```python
from build123d import *

# Parameters (mm, degrees)
BOSS_EXTRUDE1_DEPTH = 20
SKETCH2_R           = 4.835
BOSS_EXTRUDE2_DEPTH = 4
CUT_EXTRUDE1_REACH  = 64.738
SKETCH3_R           = 7.665
CUT_EXTRUDE2_DEPTH  = 10
SKETCH5_W           = 6
SKETCH5_H           = 4
CUT_EXTRUDE3_DEPTH  = 10
CUT_EXTRUDE4_REACH  = 64.738
SKETCH6_R           = 1.165
BOSS_EXTRUDE4_DEPTH = 4
BOSS_EXTRUDE5_START = -4
BOSS_EXTRUDE5_DEPTH = 4
CHAMFER1_SIZE       = 3
CHAMFER2_SIZE       = 1
CHAMFER3_SIZE       = 1


with BuildPart() as part:
    # Sketch1 → Boss-Extrude1 (new body)
    with BuildSketch(Plane.XY):
        Polygon((-40.25, -10), (-40.25, -6), (-50, -6), (-56, -6), (-56, 6), (-50, 6), (-40.25, 6), (-40.25, 10), (0, 10), (2.25, 10), (2.25, 6), (0, 6), (-9.75, 6), (-9.75, -6), (0, -6), (2.25, -6), (2.25, -10), (0, -10), align=None)
    extrude(amount=BOSS_EXTRUDE1_DEPTH)

    # Sketch2 → Boss-Extrude2 (add)
    with BuildSketch(Plane.XZ.offset(6)):
        with Locations(Location((-50, 10, 0), (0, 0, 180))):
            Circle(SKETCH2_R)
    boss_extrude2 = extrude(amount=BOSS_EXTRUDE2_DEPTH)

    # Cut-Extrude1: up to this face of the body (flat: up to its plane)
    cut_extrude1_end = Plane(part.part.faces().sort_by_distance((-19, 10, 10))[0])
    # Sketch3 → Cut-Extrude1 (cut, up to the picked face)
    with BuildSketch(Plane.XZ.offset(10), mode=Mode.PRIVATE) as cut_extrude1_sk1:
        with Locations((0, 10)):
            Circle(SKETCH3_R)
    cut_extrude1_tool1 = split(extrude(cut_extrude1_sk1.sketch, amount=-CUT_EXTRUDE1_REACH, mode=Mode.PRIVATE), bisect_by=cut_extrude1_end, keep=Keep.BOTH, mode=Mode.PRIVATE)
    add(cut_extrude1_tool1.solids().sort_by(Axis((0, -10, 10), (0, 1, 0)))[0], mode=Mode.SUBTRACT)

    # Mirror1: Boss-Extrude2 across plane
    add(boss_extrude2.mirror(Plane.ZX))

    # Sketch4 → Cut-Extrude2 (cut)
    with BuildSketch(Plane.XY.offset(20)):
        Polygon((-27.5, 2.5), (-22.5, 2.062556682), (-22.5, -2.062556682), (-27.5, -2.5), align=None)
    extrude(amount=-CUT_EXTRUDE2_DEPTH, mode=Mode.SUBTRACT)

    # Sketch5 → Cut-Extrude3 (cut)
    with BuildSketch(Plane.XY.offset(20)):
        with Locations((-30.5, 5.165)):
            Rectangle(SKETCH5_W, SKETCH5_H)
        with Locations((-19.5, 5.165)):
            Rectangle(SKETCH5_W, SKETCH5_H)
        with Locations((-19.5, -5.165)):
            Rectangle(SKETCH5_W, SKETCH5_H)
        with Locations((-30.5, -5.165)):
            Rectangle(SKETCH5_W, SKETCH5_H)
    extrude(amount=-CUT_EXTRUDE3_DEPTH, mode=Mode.SUBTRACT)

    # Cut-Extrude4: up to this face of the body (flat: up to its plane)
    cut_extrude4_end = Plane(part.part.faces().sort_by_distance((-21.952820108, 10, 10))[0])
    # Sketch6 → Cut-Extrude4 (cut, up to the picked face)
    with BuildSketch(Plane.XZ.offset(10), mode=Mode.PRIVATE) as cut_extrude4_sk1:
        with Locations(Location((-30.5, 13, 0), (0, 0, 270))):
            Circle(SKETCH6_R)
    cut_extrude4_tool1 = split(extrude(cut_extrude4_sk1.sketch, amount=-CUT_EXTRUDE4_REACH, mode=Mode.PRIVATE), bisect_by=cut_extrude4_end, keep=Keep.BOTH, mode=Mode.PRIVATE)
    # Sketch6 → Cut-Extrude4 (cut, up to the picked face)
    with BuildSketch(Plane.XZ.offset(10), mode=Mode.PRIVATE) as cut_extrude4_sk2:
        with Locations((-25, 13)):
            Circle(SKETCH6_R)
    cut_extrude4_tool2 = split(extrude(cut_extrude4_sk2.sketch, amount=-CUT_EXTRUDE4_REACH, mode=Mode.PRIVATE), bisect_by=cut_extrude4_end, keep=Keep.BOTH, mode=Mode.PRIVATE)
    # Sketch6 → Cut-Extrude4 (cut, up to the picked face)
    with BuildSketch(Plane.XZ.offset(10), mode=Mode.PRIVATE) as cut_extrude4_sk3:
        with Locations(Location((-19.5, 13, 0), (0, 0, 90))):
            Circle(SKETCH6_R)
    cut_extrude4_tool3 = split(extrude(cut_extrude4_sk3.sketch, amount=-CUT_EXTRUDE4_REACH, mode=Mode.PRIVATE), bisect_by=cut_extrude4_end, keep=Keep.BOTH, mode=Mode.PRIVATE)
    add(cut_extrude4_tool1.solids().sort_by(Axis((-30.5, -10, 13), (0, 1, 0)))[0], mode=Mode.SUBTRACT)
    add(cut_extrude4_tool2.solids().sort_by(Axis((-25, -10, 13), (0, 1, 0)))[0], mode=Mode.SUBTRACT)
    add(cut_extrude4_tool3.solids().sort_by(Axis((-19.5, -10, 13), (0, 1, 0)))[0], mode=Mode.SUBTRACT)

    # Sketch10 → Boss-Extrude4 (add)
    with BuildSketch(Plane.XZ.offset(10)):
        with BuildLine():
            Line((2.25, 17.327327275), (3.717710372, 22.107058049))
            ThreePointArc((3.717710372, 22.107058049), (-12.665, 10), (3.717710372, -2.107058049))
            Line((3.717710372, -2.107058049), (2.25, 2.672672725))
            ThreePointArc((2.25, 2.672672725), (-7.665, 10), (2.25, 17.327327275))
        make_face()
    extrude(amount=-BOSS_EXTRUDE4_DEPTH)

    # Sketch11 → Boss-Extrude5 (add)
    with BuildSketch(Plane(origin=(0, 10, 0), x_dir=(1, 0, 0), z_dir=(0, 1, 0)).offset(BOSS_EXTRUDE5_START)):
        with BuildLine():
            Line((-9.75, -20), (-7.771886837, -20))
            ThreePointArc((-7.771886837, -20), (-2.284515289, -22.457255512), (3.717710372, -22.107058049))
            Line((3.717710372, -22.107058049), (2.25, -17.327327275))
            ThreePointArc((2.25, -17.327327275), (-7.665, -10), (2.25, -2.672672725))
            Line((2.25, -2.672672725), (3.717710372, 2.107058049))
            ThreePointArc((3.717710372, 2.107058049), (-2.284515289, 2.457255512), (-7.771886837, 0))
            Line((-7.771886837, 0), (-9.75, 0))
            Line((-9.75, 0), (-9.75, -20))
        make_face()
    extrude(amount=BOSS_EXTRUDE5_DEPTH)

    # Chamfer1
    # the kernel refuses this chamfer: 3 mm, written as the material it takes off along each edge
    with BuildSketch(Plane(origin=(-30.5, -10, 13), x_dir=(0, 0, -1), z_dir=(-1, 0, 0))) as chamfer1_piece_1:
        Polygon((1.165, -CHAMFER1_SIZE), (1.165 + CHAMFER1_SIZE, 0), (1.165, 0), align=None)
    revolve(axis=Axis((-30.5, -10, 13), (0, -1, 0)), mode=Mode.SUBTRACT)
    with BuildSketch(Plane(origin=(-25, -10, 13), x_dir=(1, 0, 0), z_dir=(0, 0, -1))) as chamfer1_piece_2:
        Polygon((1.165, -CHAMFER1_SIZE), (1.165 + CHAMFER1_SIZE, 0), (1.165, 0), align=None)
    revolve(axis=Axis((-25, -10, 13), (0, -1, 0)), mode=Mode.SUBTRACT)
    with BuildSketch(Plane(origin=(-19.5, -10, 13), x_dir=(0, 0, 1), z_dir=(1, 0, 0))) as chamfer1_piece_3:
        Polygon((1.165, -CHAMFER1_SIZE), (1.165 + CHAMFER1_SIZE, 0), (1.165, 0), align=None)
    revolve(axis=Axis((-19.5, -10, 13), (0, -1, 0)), mode=Mode.SUBTRACT)

    # Chamfer2
    chamfer2_edges = [part.edges().sort_by_distance(p)[0] for p in [
        (-45.165, -10, 10),
    ]]
    chamfer(chamfer2_edges, length=CHAMFER2_SIZE)

    # Chamfer3
    chamfer3_edges = [part.edges().sort_by_distance(p)[0] for p in [
        (-45.165, 10, 10),
    ]]
    chamfer(chamfer3_edges, length=CHAMFER3_SIZE)


solid = part.part
```
Check sheet for the modelled part. Datum: model origin and axes. Units: mm. A direction names the side the tool comes from. Give positions to 0.01 mm unless a question says otherwise; leave off trailing zeros. Order: outer loops, then holes, each group sorted by start corner. A loop starts at its lowest first (then second) coordinate and runs counter-clockwise, first axis right, second up. Notation, with made-up numbers: (77, 44.25) -> (134, 44.25) arc R35 cw to (134, 78.25) -> close; hole circle Ø3 at (27.5, 40). An arc over 180 degrees is marked (long way). Return JSON: item names as keys, results as strings.
1. Go/stop test with flat-tipped pins: P1, Ø3, axis at y = -5, z = 13, coming from the +X side; P2, Ø6, axis at x = -37.5, y = 5, coming from the -Z side; P3, Ø3, axis at x = -20.5, y = -6, coming from the +Z side. Record where each tip stops, or that it passes through.
From the geometry:
{"P1": "x = -6.46", "P2": "z = 0", "P3": "z = 20"}
2. Mould release check, pull along X, two halves, no side actions. Record for faces 1 (the cylindrical face through (-2.201, -8.028, 22.472)), 2 (the flat face through (2.994, 7.972, 19.751)), 3 (the cylindrical face through (-18.791, -0.044, 12.075)): +X half, -X half, draft (parallel to the pull), parting line (faces both ways), or undercut.
From the geometry:
{"face 1": "parting line", "face 2": "+X half", "face 3": "undercut"}
3. Material ranges on probe 1 along X at (y, z) = (5, 13) (3 decimals); probe 2 along X at (y, z) = (-5, 15.5); probe 3 along X at (y, z) = (-1, 13) (3 decimals), recorded low to high. Write a range as [from, to].
From the geometry:
{"probe 1": "[-56, -33.5], [-27.5, -26.165], [-23.835, -22.5], [-16.5, -9.75]", "probe 2": "[-56, -33.5], [-27.5, -22.5], [-16.5, -9.75]", "probe 3": "[-56, -31.665], [-29.335, -27.5], [-22.5, -20.665], [-18.335, -9.75]"}
4. Cross-section at B-B, the plane x = 0. Record the cut outline in (y, z) (3 decimals), plus the area to 3 significant figures.
From the geometry:
{"outline": "(-10, -2.665) -> (-6, -2.665) -> (-6, 2.335) -> (-10, 2.335) -> close; (-10, 17.665) -> (-6, 17.665) -> (-6, 22.665) -> (-10, 22.665) -> close; (6, -2.665) -> (10, -2.665) -> (10, 2.335) -> (6, 2.335) -> close; (6, 17.665) -> (10, 17.665) -> (10, 22.665) -> (6, 22.665) -> close", "area": "80.0 mm^2"}
5. Cross-section at A-A, the plane y = 8. Record the cut outline in (x, z) (3 decimals), plus the area to 3 significant figures.
From the geometry:
{"outline": "circle Ø9.67 at (-50, 10); (-40.25, 0) -> (-7.772, 0) arc R12.665 ccw to (3.718, -2.107) -> (2.25, 2.673) arc R7.665 cw (long way) to (2.25, 17.327) -> (3.718, 22.107) arc R12.665 ccw to (-7.772, 20) -> (-40.25, 20) -> close; hole circle Ø2.33 at (-30.5, 13); hole circle Ø2.33 at (-25, 13); hole circle Ø2.33 at (-19.5, 13)", "area": "832 mm^2"}
6. Cross-section at D-D, the plane x = -30.5. Record the cut outline in (y, z) (3 decimals), plus the area to 3 significant figures.
From the geometry:
{"outline": "(-10, 0) -> (10, 0) -> (10, 11.835) -> (7.165, 11.835) -> (7.165, 10) -> (3.165, 10) -> (3.165, 11.835) -> (-3.165, 11.835) -> (-3.165, 10) -> (-7.165, 10) -> (-7.165, 11.67) -> (-10, 8.835) -> close; (-10, 17.165) -> (-7.165, 14.33) -> (-7.165, 20) -> (-10, 20) -> close; (-3.165, 14.165) -> (3.165, 14.165) -> (3.165, 20) -> (-3.165, 20) -> close; (7.165, 14.165) -> (10, 14.165) -> (10, 20) -> (7.165, 20) -> close", "area": "283 mm^2"}
7. Cross-section at C-C, the plane y = 1.25. Record the cut outline in (x, z) (3 decimals), plus the area to 3 significant figures.
From the geometry:
{"outline": "(-56, 0) -> (-9.75, 0) -> (-9.75, 20) -> (-22.5, 20) -> (-22.5, 10) -> (-27.5, 10) -> (-27.5, 20) -> (-56, 20) -> close; hole circle Ø2.33 at (-30.5, 13); hole circle Ø2.33 at (-19.5, 13)", "area": "866 mm^2"}
8. Set-up check for faces 4 (the cylindrical face through (-45.17, -7.48, 9.79)), 5 (the flat face through (-26, 0, 0)), 6 (the cylindrical face through (-24.462, -4.623, 11.966)), 7 (the flat face through (-25, 0, 10)): record each of +Z, -Z, +X, -X, +Y, -Y from which the full face is reachable in a straight line by a thin tool's end or side.
From the geometry:
{"face 4": "-Y", "face 5": "-Z, -X, +Y, -Y", "face 6": "+Y, -Y", "face 7": "+Z"}
